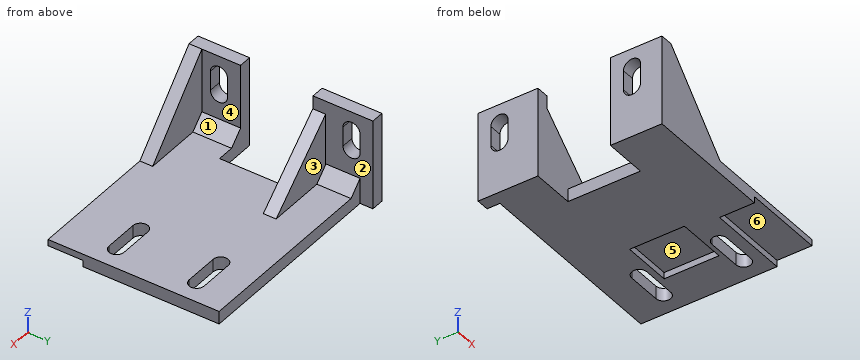
Autodesk Inventor part; units mm, degrees
ref_plane "YZ Plane" through (0, 0, 0) normal (1, 0, 0) x (0, 1, 0)
ref_plane "XZ Plane" through (0, 0, 0) normal (0, 1, 0) x (-1, 0, 0)
ref_plane "XY Plane" through (0, 0, 0) normal (0, 0, 1) x (1, 0, 0)
sketch "Sketch1" plane through (0, 0, 0) normal (0, 0, 1) x (1, 0, 0)
  line L0 (0, 0) -> (50, 0)
  line L1 (50, 0) -> (50, -40)
  line L2 (50, -40) -> (0, -40)
  line L3 (0, -40) -> (0, 0)
  dimension "d0" = 50
  dimension "d1" = 40
extrude "Extrusion1" add sketch "Sketch1" along normal blind 3
sketch "Sketch2" plane through (0, 0, 3) normal (0, 0, 1) x (1, 0, 0)
  line L0 (0, -40) -> (50, -40)
  line L1 (0, 0) -> (3, 0)
  line L2 (3, 0) -> (3, -40)
  line L3 (3, -40) -> (0, -40)
  line L4 (0, -40) -> (0, 0)
  dimension "d4" = 3
extrude "Extrusion2" add sketch "Sketch2" along normal blind 18
sketch "Sketch3" plane through (0, 0, 0) normal (0, 1, 0) x (1, 0, 0)
  line L0 (0, 0) -> (3, 0)
  line L1 (3, 0) -> (3, -21)
  line L2 (3, -21) -> (0, -21)
  line L3 (0, -21) -> (0, 0)
extrude "Extrusion3" add sketch "Sketch3" along normal blind 3
sketch "Sketch4" plane through (0, 0, 0) normal (0, 0, -1) x (-1, 0, 0)
  line L0 (0, -40) -> (0, 3)
  line L1 (-3, 0) -> (-3, 3)
  line L2 (-3, 0) -> (-3, -11)
  line L3 (0, -11) -> (-10, -11)
  line L4 (-10, -11) -> (-10, -27.9486)
  line L5 (-10, -27.9486) -> (0, -27.9486)
  point P0 (0, 0)
  dimension "d9" = 11
  dimension "d10" = 10
extrude "Extrusion4" cut sketch "Sketch4" against normal blind 8
sketch "Sketch6" plane through (0, -40, 0) normal (-1, 0, 0) x (0, 0, 1)
  line L0 (0, 29) -> (8, 29)
  line L1 (12, 38) -> (16.5475, 38) construction
  line L2 (12, 36) -> (16.5475, 36)
  line L3 (16.5475, 40) -> (12, 40)
  arc A0 (12, 40) -> (12, 36) centre (12, 38) ccw
  arc A1 (16.5475, 36) -> (16.5475, 40) centre (16.5475, 38) ccw
  point P0 (0, 40)
  point P1 (14.2738, 38)
extrude "Extrusion6" cut sketch "Sketch6" against normal through all
sketch "Sketch7" plane through (0, -40, 0) normal (-1, 0, 0) x (0, 0, 1)
  line L0 (16.5475, 36) -> (12, 36)
  line L1 (12, 7) -> (16.5475, 7) construction
  line L2 (12, 5) -> (16.5475, 5)
  line L3 (16.5475, 9) -> (12, 9)
  arc A0 (12, 9) -> (12, 5) centre (12, 7) ccw
  arc A1 (16.5475, 5) -> (16.5475, 9) centre (16.5475, 7) ccw
  point P0 (0, 40)
  point P1 (14.2738, 7)
  dimension "d67" = 4
extrude "Extrusion7" cut sketch "Sketch7" against normal through all
sketch "Sketch8" plane through (0, 0, 0) normal (0, 0, -1) x (-1, 0, 0)
  line L0 (-45, -8.75) -> (-37, -8.75) construction
  line L1 (-45, -10.5) -> (-37, -10.5)
  line L2 (-37, -7) -> (-45, -7)
  arc A0 (-45, -7) -> (-45, -10.5) centre (-45, -8.75) ccw
  arc A1 (-37, -10.5) -> (-37, -7) centre (-37, -8.75) ccw
  line L3 (-10, -27.9486) -> (-10, -11)
  line L4 (-41, -8.75) -> (-41, -4.75) construction
  line L5 (-41, -4.75) -> (-35.5779, -4.75) construction
  point P0 (0, 0)
  dimension "d27" = 8
  dimension "d28" = 3.5
  dimension "d60" = 4
extrude "Extrusion8" cut sketch "Sketch8" against normal through all
chamfer "Chamfer1" distance 3 angle 45 1 edges at (3, -33.9743, 3)
chamfer "Chamfer2" distance 3 angle 45 1 edges at (3, -5.5, 3)
sketch "Sketch11" plane through (0, 0, 0) normal (0, 0, -1) x (-1, 0, 0)
  line L0 (-10, -27.9486) -> (-10, -11)
  line L1 (-41.0188, 5.0018) -> (-41.0188, -13.9982) construction
  line L2 (-48.6932, -22.9665) -> (-25.0226, -22.9665) construction
  line L3 (-45, -41.7147) -> (-45, -21.8236) construction
  line L4 (-37, -41.7147) -> (-37, -21.8236) construction
  line L5 (-45, -22.9665) -> (-37, -22.9665) construction
  line L6 (-45, -29.2482) -> (-37, -29.2482)
  arc A0 (-45, -25.7482) -> (-45, -29.2482) centre (-45, -27.4982) ccw
  arc A1 (-37, -29.2482) -> (-37, -25.7482) centre (-37, -27.4982) ccw
  line L7 (0, -27.9486) -> (-10, -27.9486)
  line L8 (-41.0188, -8.7165) -> (-41.0188, -4.7165)
  line L9 (-41.0188, -4.7165) -> (-38.5918, -4.7165)
  line L10 (0, -40) -> (0, -27.9486)
  line L11 (-41.0188, 5.7518) -> (-41.0188, -13.2482) construction
  line L12 (-41.0188, -27.7165) -> (-56.6295, -27.7165) construction
  line L13 (-37, -25.7482) -> (-45, -25.7482)
  point P0 (0, 0)
  point P1 (-41, -22.9665)
  dimension "d43" = 19
  dimension "d44" = 3.5
  dimension "d59" = 4
  dimension "d61" = 19
extrude "Extrusion11" cut sketch "Sketch11" against normal through all
sketch "Sketch12" plane through (0, 0, 0) normal (0, 0, -1) x (-1, 0, 0)
  line L0 (-10, -27.9486) -> (-10, -11)
  line L1 (-41, -25.8493) -> (-41, -31.8493) construction
  line L2 (-41, -31.8493) -> (-30.8265, -31.8493) construction
  line L3 (-30.8265, -31.8493) -> (-30.8265, -35.8493) construction
  line L4 (-30.8265, -35.8493) -> (-30.8265, -31.8493) construction
  line L5 (-30.8265, -31.8493) -> (-50, -31.8493)
  line L6 (-50, -31.8493) -> (-50, -40)
  line L7 (-50, -40) -> (-30.8265, -40)
  line L8 (-30.8265, -40) -> (-30.8265, -31.8493)
  point P0 (0, 0)
  dimension "d47" = 6
  dimension "d48" = 4
  dimension "d49" = 4
extrude "Extrusion12" cut sketch "Sketch12" against normal blind 1.5
sketch "Sketch13" plane through (0, 0, 0) normal (0, 0, -1) x (-1, 0, 0)
  line L0 (-45, -21.2165) -> (-37, -21.2165)
  arc A0 (-37, -10.5) -> (-37, -7) centre (-37, -8.75) ccw
  arc A1 (-45, -7) -> (-45, -10.5) centre (-45, -8.75) ccw
  line L1 (-45, -7) -> (-37, -7)
  line L2 (-46.75, -8.75) -> (-40.75, -8.75) construction
  line L3 (-40.75, -8.75) -> (-40.75, -24.7606) construction
  line L4 (-40.75, -24.7606) -> (-37.75, -24.7606) construction
  line L5 (-37.75, -11.2484) -> (-40.75, -11.2484) construction
  line L6 (-35.25, -8.75) -> (-29.25, -8.75) construction
  line L7 (-29.25, -8.75) -> (-29.25, -11.925) construction
  line L8 (-40.8665, -21.2165) -> (-40.75, -19.2199) construction
  line L9 (-29.25, -11.925) -> (-40.75, -11.925)
  line L10 (-40.75, -11.925) -> (-40.75, -24.7606)
  line L11 (-40.75, -24.7606) -> (-29.25, -24.7606)
  line L12 (-29.25, -24.7606) -> (-29.25, -11.925)
  point P0 (0, 0)
  point P1 (-40.75, -11.925)
  dimension "d52" = 6
  dimension "d53" = 3
  dimension "d54" = 6
  dimension "d55" = 3.175
  dimension "d56" = 2
extrude "Extrusion13" cut sketch "Sketch13" against normal blind 1.5
ref_plane "Work Plane1" through (0, -8, 0) normal (0, 1, 0) x (1, 0, 0)
sketch "Sketch14" plane through (0, -8, 0) normal (0, 1, 0) x (1, 0, 0)
  line L0 (3.0794, -17.957) -> (19.7008, -2.8939)
  line L1 (19.7008, -2.8939) -> (3.0794, -2.8939)
  line L2 (3.0794, -2.8939) -> (3.0794, -17.957)
  point P0 (0, 0)
extrude "Extrusion14" add sketch "Sketch14" against normal blind 3
sketch "Sketch15" plane through (0, -40, 21) normal (0, -1, 0) x (1, 0, 0)
  line L0 (6, -18) -> (50, -18)
  line L1 (3, -15) -> (6, -18)
  line L2 (3, -15) -> (3, 0)
  line L3 (3, 0) -> (19.3977, -18)
  line L4 (3, -15.75) -> (3, 0)
extrude "Extrusion15" add sketch "Sketch15" against normal blind 3
sketch "Sketch16" plane through (3, 0, 0) normal (1, 0, 0) x (0, 0, -1)
  line L0 (-21, -37) -> (-21, 3)
  line L1 (-21, -11) -> (-8, -11)
  line L2 (-8, -11) -> (-8, -27.9486)
  line L3 (-8, -27.9486) -> (-21, -27.9486)
  line L4 (-21, -27.9486) -> (-21, -11)
extrude "Extrusion16" cut sketch "Sketch16" against normal through all
properties part number "bart z endstop bracket v12"
Input: part model. Units: mm. Frame: model coordinates. Face numbers are marked on the shaded views. A direction names the side the tool comes from. Coordinates: 2 decimals unless noted, no trailing zeros. Loops run counter-clockwise (first coordinate to the right, second up) from the corner with the lowest first, then second, coordinate; pieces in that order, holes last.
Q1. Contact query for flat-ended pins moving along their axis: pin 1 (12 mm diameter, centred on y = -18, z = 11, fed in from -X); pin 2 (0.8 mm diameter, centred on x = 34, z = 1, fed in from -Y); pin 3 (6 mm diameter, centred on y = -3.5, z = 18, fed in from +X); pin 4 (12 mm diameter, centred on x = 26, y = -26.5, fed in from +Z). Output: stop coordinate, or through.
Q2. Set-up query: the marked faces 4, 5 and 6. Return all of +Z, -Z, +X, -X, +Y, -Y with unobstructed straight access to the full face (end or side cutting, diameter ignored); none if empty.
Q3. Cut plane D-D (x = 16). Output: boundary loops of the cut face in (y, z).
Q4. Cut plane A-A (y = -33). Output: boundary loops of the cut face in (x, z), then the cut area to 3 significant figures.
Q5. Draft query along X for the marked faces 1, 2 and 3. Return one class per face: +X half, -X half, draft (parallel to the pull), parting line (faces both ways), or undercut.
Q6. Cut plane C-C (z = 14.5). Output: boundary loops of the cut face in (x, y).
Q7. Cut plane B-B (y = -24). Output: boundary loops of the cut face in (x, z), then the cut area to 3 significant figures.
Q8. Material intervals for line 1 (Y direction, x = 8, z = 12.5); line 2 (Z direction, x = 41, y = -24.5), sorted ascending.
Working result:
1. pin 1: passes through
1. pin 2: stops at y = -31.85
1. pin 3: stops at x = 3
1. pin 4: stops at z = 3
2. face 4: +Z, +X, +Y
2. face 5: -Z
2. face 6: -Z, +X, -Y
3. outline: (-40, 0) - (0, 0) - (0, 3) - (-8, 3) - (-8, 6.25) - (-11, 6.25) - (-11, 3) - (-37, 3) - (-37, 6.73) - (-40, 6.73) - close
4. outline: (0, 0) - (30.83, 0) - (30.83, 1.5) - (50, 1.5) - (50, 3) - (6, 3) - (3, 6) - (3, 10) - (0, 10) - close; (0, 18.55) - (3, 18.55) - (3, 21) - (0, 21) - close
4. area: 154 mm2
5. face 1: +X half
5. face 2: undercut
5. face 3: draft
6. outline: (0, -40) - (8.92, -40) - (8.92, -37) - (3, -37) - (3, -35) - (0, -35) - close; (0, -31) - (3, -31) - (3, -27.95) - (0, -27.95) - close; (0, -11) - (3, -11) - (3, -4) - (0, -4) - close; (0, 0) - (3, 0) - (3, 3) - (0, 3) - close; (3.08, -11) - (6.89, -11) - (6.89, -8) - (3.08, -8) - close
7. outline: (10, 0) - (29.25, 0) - (29.25, 1.5) - (40.75, 1.5) - (40.75, 0) - (50, 0) - (50, 3) - (10, 3) - close
7. area: 103 mm2
8. line 1: y = -40 to -37, -11 to -8
8. line 2: z = 0 to 3
